from build123d import *

# Parameters (mm, degrees)
BOSS_EXTRU_1_DEPTH      = 2
CONG_1_R                = 2
BOSS_EXTRU_2_DEPTH      = 8
ENL_V_MAT_EXTRU_1_DEPTH = 5


with BuildPart() as part:
    # Esquisse1 → Boss.-Extru.1 (new body)
    with BuildSketch(Plane(origin=(0, 0, 0), x_dir=(1, 0, 0), z_dir=(0, 1, 0))):
        with BuildLine():
            Line((0, 4.5), (6.5, 4.5))
            ThreePointArc((6.5, 4.5), (11, 0), (6.5, -4.5))
            Line((6.5, -4.5), (0, -4.5))
            ThreePointArc((0, -4.5), (-4.5, 0), (0, 4.5))
        make_face()
    extrude(amount=BOSS_EXTRU_1_DEPTH)

    # Congé1
    cong_1_edges = [part.edges().sort_by_distance(p)[0] for p in [
        (3.25, 0, -4.5),
        (11, 0, 0),
        (-4.5, 0, 0),
        (3.25, 0, 4.5),
    ]]
    fillet(cong_1_edges, radius=CONG_1_R - 0.0001)  # a hair under: the kernel refuses the full size

    # Esquisse2 → Boss.-Extru.2 (add)
    with BuildSketch(Plane(origin=(0, 2, 0), x_dir=(1, 0, 0), z_dir=(0, 1, 0))):
        Polygon((-2.75, -2.75), (9.25, -2.75), (9.25, -1.5), (10.5, -1.5), (10.5, 1.5), (9.25, 1.5), (9.25, 2.75), (-2.75, 2.75), (-2.75, 1.5), (-4, 1.5), (-4, -1.5), (-2.75, -1.5), align=None)
    extrude(amount=BOSS_EXTRU_2_DEPTH)

    # Esquisse4 → Enlèv. mat.-Extru.1 (cut)
    with BuildSketch(Plane.XZ):
        with BuildLine():
            Line((6.5, 1.5), (0, 1.5))
            ThreePointArc((0, 1.5), (-1.5, 0), (0, -1.5))
            Line((0, -1.5), (6.5, -1.5))
            ThreePointArc((6.5, -1.5), (8, 0), (6.5, 1.5))
        make_face()
    extrude(amount=-ENL_V_MAT_EXTRU_1_DEPTH, mode=Mode.SUBTRACT)


solid = part.part
Geometry check sheet. Reference: the model listing, model coordinates, mm. A direction names the side the tool comes from. Give positions to 0.01 mm unless a question says otherwise; leave off trailing zeros. Order: outer loops, then holes, each group sorted by start corner. A loop starts at its lowest first (then second) coordinate and runs counter-clockwise, first axis right, second up. Notation, with made-up numbers: (40.25, 32) - (62.25, 32) arc R36 ccw to (62.25, 68) - close; hole circle Ø2 at (30.25, 52.5). An arc over 180 degrees is marked (long way). Answer as a JSON object with one key per item and string values.
(1) Cross-section at C-C (y = 7.5). Record the cut outline in (x, z), then the cut area to 3 significant figures.
Report:
{"outline": "(-4, -1.5) - (-2.75, -1.5) - (-2.75, -2.75) - (9.25, -2.75) - (9.25, -1.5) - (10.5, -1.5) - (10.5, 1.5) - (9.25, 1.5) - (9.25, 2.75) - (-2.75, 2.75) - (-2.75, 1.5) - (-4, 1.5) - close", "area": "73.5 mm^2"}
(2) Depth check by flat-ended pin: pin 1 Ø0.9 at (y, z) = (4.5, -0.5) entering from +X; pin 2 Ø2.5 at (y, z) = (5, 0) entering from -X; pin 3 Ø1 at (x, y) = (-3, 6.5) entering from +Z; pin 4 Ø3 at (x, y) = (-0.5, 2) entering from -Z. Enter the tip coordinate at first touch or a pass-through.
Report:
{"pin 1": "x = 10.5", "pin 2": "x = -4", "pin 3": "z = 2.75", "pin 4": "z = -4.5"}
(3) Tool access check on faces 1 (the flat face through (-3, 6, -1.5)), 2 (the flat face through (3, 6, -2.75)), 3 (the cylindrical face through (-1.5, 2.5, 0)), 4 (the flat face through (10, 6, 1.5)). Record the directions out of +Z, -Z, +X, -X, +Y, -Y that give a thin tool (end or side, any length) a straight path to the whole face; none if there is none.
Report:
{"face 1": "-Z, -X, +Y", "face 2": "-Z, +X, -X, +Y", "face 3": "-Y", "face 4": "+Z, +X, +Y"}
(4) Draft check along Z on faces 5 (the flat face through (3, 5, 0)), 6 (the flat face through (10, 6, -1.5)), 7 (the flat face through (-4, 6, 0)). Enter one of: released by +Z, released by -Z, zero draft, split by the parting line, or undercut.
Report:
{"face 5": "undercut", "face 6": "released by -Z", "face 7": "zero draft"}
(5) Material ranges on line 1 (Y direction, x = 0.25, z = -0.5); line 2 (X direction, y = 8.75, z = 0); line 3 (Z direction, x = -2.5, y = 4.25), recorded low to high.
Report:
{"line 1": "5 to 10", "line 2": "-4 to 10.5", "line 3": "-2.75 to 2.75"}
